The model under review builds one solid part; all positions refer to its coordinate system, in mm. A direction names the side the tool comes from. Coordinates: 2 decimals unless noted, no trailing zeros. Order: outer loops, then holes, each group sorted by start corner. A loop starts at its lowest first (then second) coordinate and runs counter-clockwise, first axis right, second up. Notation, with made-up numbers: M -29,19 L 29,19 A30 cw 29,45 Z; hole C -17.5,-27 d2. An arc over 180 degrees is marked long. One line per item, written item: value.
```python
from build123d import *

# Parameters (mm, degrees)
BOSS_EXTRUDE1_DEPTH = 15
ESQUISSE1_W         = 12
ESQUISSE1_H         = 10
BOSS_EXTRU_1_DEPTH  = 9
ESQUISSE2_R         = 2.5
BOSS_EXTRU_2_DEPTH  = 2
BOSS_EXTRUDE2_DEPTH = 10


with BuildPart() as part:
    # Sketch1 → Boss-Extrude1 (new body)
    with BuildSketch(Plane.XY):
        with BuildLine():
            Line((-3.31662479, 5), (3.31662479, 5))
            ThreePointArc((3.31662479, 5), (6, 0), (3.31662479, -5))
            Line((3.31662479, -5), (-3.31662479, -5))
            ThreePointArc((-3.31662479, -5), (-6, 0), (-3.31662479, 5))
        make_face()
    extrude(amount=BOSS_EXTRUDE1_DEPTH)

    # Esquisse1 → Boss.-Extru.1 (add)
    with BuildSketch(Plane.XY.offset(15)):
        Rectangle(ESQUISSE1_W, ESQUISSE1_H)
    extrude(amount=BOSS_EXTRU_1_DEPTH)

    # Esquisse2 → Boss.-Extru.2 (add)
    with BuildSketch(Plane(origin=(0, 0, 0), x_dir=(-1, 0, 0), z_dir=(0, 0, -1))):
        Circle(ESQUISSE2_R)
    extrude(amount=BOSS_EXTRU_2_DEPTH)

    # Sketch2 → Boss-Extrude2 (add)
    with BuildSketch(Plane.XY.offset(24)):
        with BuildLine():
            Line((-1.118033989, 1), (1.118033989, 1))
            ThreePointArc((1.118033989, 1), (0, -1.5), (-1.118033989, 1))
        make_face()
    extrude(amount=BOSS_EXTRUDE2_DEPTH)


solid = part.part
```
(1) Tool access review of faces 1 (the flat face through (-5, -4, 15)), 2 (the flat face through (-5, 4, 15)), 3 (the cylindrical face through (6, 0, 7)), 4 (the cylindrical face through (0, -1.5, 28.9)): name each direction out of +Z, -Z, +X, -X, +Y, -Y from which nothing blocks a thin tool from reaching the whole face with its end or side.
Geometry results:
face 1: -Z, -X, -Y
face 2: -Z, -X, +Y
face 3: -Z, +X
face 4: +Z
(2) We need section D-D, the plane y = -2. State the section outline as (x, z) points, plus the area to 3 significant figures.
Geometry results:
outline: M -6,15 L -5.66,15 L -5.66,0 L -1.5,0 L -1.5,-2 L 1.5,-2 L 1.5,0 L 5.66,0 L 5.66,15 L 6,15 L 6,24 L -6,24 Z
area: 284 mm2
(3) We need section C-C, the plane z = 5.5. State the section outline as (x, y) points.
Geometry results:
outline: M -3.32,-5 L 3.32,-5 A6 ccw 3.32,5 L -3.32,5 A6 ccw Z
(4) We need section A-A, the plane x = 0. State the section outline as (y, z) points, plus the area to 3 significant figures.
Geometry results:
outline: M -5,0 L -2.5,0 L -2.5,-2 L 2.5,-2 L 2.5,0 L 5,0 L 5,24 L 1,24 L 1,34 L -1.5,34 L -1.5,24 L -5,24 Z
area: 275 mm2
(5) Insertion check: pin 1 Ø2 at (y, z) = (0.5, 27.5) entering from +X; pin 2 Ø3 at (x, y) = (-4.5, 3) entering from -Z; pin 3 Ø0.7 at (x, z) = (0.5, 28.5) entering from +Y. Each pin has a flat end and moves straight along its axis. Give the tip position at first contact, or say it passes through.
Geometry results:
pin 1: stops at x = 1.5
pin 2: stops at z = 0
pin 3: stops at y = 1
(6) For L1, parallel to Z at x = -1, y = 1.75; L2, parallel to Y at x = -1, z = 26; L3, parallel to Z at x = -4.75, y = 2.5, list the stretches that pass through material, from the lowest coordinate up.
Geometry results:
L1: z = -2 to 24
L2: y = -1.12 to 1
L3: z = 0 to 24
